Can you work these out from the model? Positions are in its coordinate system, mm. Face numbers are marked on the shaded views. A direction names the side the tool comes from. Give positions to 0.01 mm unless a question says otherwise; leave off trailing zeros. Write each loop counter-clockwise with the first axis right and the second up, starting at its lowest first coordinate (ties: lowest second). Pieces come first, ordered by that corner, then holes. Notation, with made-up numbers: M 85.25,62.25 L 140.25,62.25 A21 cw 140.25,70.25 Z; hole C 10.25,-4.5 d10. An arc over 180 degrees is marked long. Use CSV: the item, a comma, the result in double quotes. Start each with the question number.
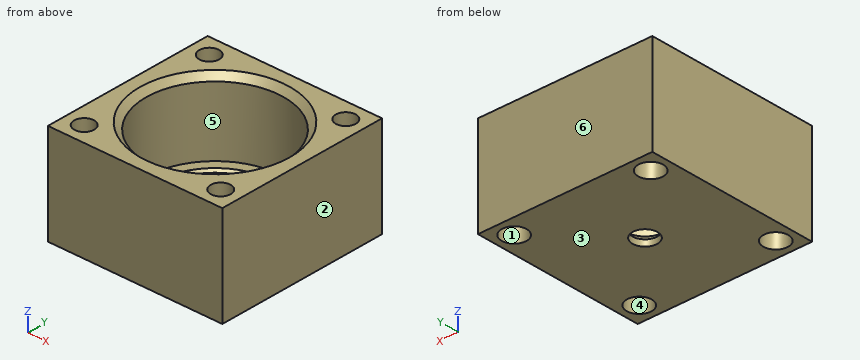
from build123d import *

# Parameters (mm, degrees)
SKETCH_W        = 28
SKETCH_H        = 28
SKETCH_R        = 2
PAD_DEPTH       = 2
SKETCH001_W     = 28
SKETCH001_H     = 28
SKETCH001_R     = 9
SKETCH001_R_2   = 2
PAD001_DEPTH    = 2
SKETCH003_W     = 28
SKETCH003_H     = 28
SKETCH003_R     = 1.6
SKETCH003_R_2   = 11
PAD002_DEPTH    = 12
CHAMFER_SIZE    = 1
CHAMFER001_SIZE = 0.4
CHAMFER002_SIZE = 1


with BuildPart() as part:
    # Sketch → Pad (new body)
    with BuildSketch(Plane.XY):
        Rectangle(SKETCH_W, SKETCH_H)
        Circle(SKETCH_R, mode=Mode.SUBTRACT)
        with Locations((10.960155, 10.960155)):
            Circle(SKETCH_R, mode=Mode.SUBTRACT)
        with Locations((-10.960155, 10.960155)):
            Circle(SKETCH_R, mode=Mode.SUBTRACT)
        with Locations((-10.960155, -10.960155)):
            Circle(SKETCH_R, mode=Mode.SUBTRACT)
        with Locations((10.960155, -10.960155)):
            Circle(SKETCH_R, mode=Mode.SUBTRACT)
    extrude(amount=PAD_DEPTH)

    # Sketch001 (on Face11 of Pad) → Pad001 (join)
    with BuildSketch(Plane.XY.offset(2)):
        Rectangle(SKETCH001_W, SKETCH001_H)
        Circle(SKETCH001_R, mode=Mode.SUBTRACT)
        with Locations((-10.960155, 10.960155)):
            Circle(SKETCH001_R_2, mode=Mode.SUBTRACT)
        with Locations((-10.960155, -10.960155)):
            Circle(SKETCH001_R_2, mode=Mode.SUBTRACT)
        with Locations((10.960155, -10.960155)):
            Circle(SKETCH001_R_2, mode=Mode.SUBTRACT)
        with Locations((10.960155, 10.960155)):
            Circle(SKETCH001_R_2, mode=Mode.SUBTRACT)
    extrude(amount=PAD001_DEPTH)

    # Sketch003 (on Face14 of Pad001) → Pad002 (join)
    with BuildSketch(Plane.XY.offset(4)):
        Rectangle(SKETCH003_W, SKETCH003_H)
        with Locations((-10.960155, 10.960155)):
            Circle(SKETCH003_R, mode=Mode.SUBTRACT)
        with Locations((-10.960155, -10.960155)):
            Circle(SKETCH003_R, mode=Mode.SUBTRACT)
        with Locations((10.960155, -10.960155)):
            Circle(SKETCH003_R, mode=Mode.SUBTRACT)
        with Locations((10.960155, 10.960155)):
            Circle(SKETCH003_R, mode=Mode.SUBTRACT)
        Circle(SKETCH003_R_2, mode=Mode.SUBTRACT)
    extrude(amount=PAD002_DEPTH)

    # Chamfer
    chamfer_edges = [part.edges().sort_by_distance(p)[0] for p in [
        (-11, 0, 16),
    ]]
    chamfer(chamfer_edges, length=CHAMFER_SIZE)

    # Chamfer001
    chamfer001_edges = [part.edges().sort_by_distance(p)[0] for p in [
        (-9, 0, 4),
    ]]
    chamfer(chamfer001_edges, length=CHAMFER001_SIZE)

    # Chamfer002
    chamfer002_edges = [part.edges().sort_by_distance(p)[0] for p in [
        (-2, 0, 2),
    ]]
    chamfer(chamfer002_edges, length=CHAMFER002_SIZE)


solid = part.part
(1) Which directions (+Z, -Z, +X, -X, +Y, -Y) give clear straight access to the entire face, cutting with the end or side of a thin tool? Please do the marked faces 4, 5 and 6.
(2) Thinking about a two-plate mould opening in X: for the marked faces 1, 2 and 3, which applies, released by +X, released by -X, zero draft, split by the parting line, or undercut?
(3) I want a section at C-C (z = 8.5). Write out the boundary of the cut face in (x, y).
(4) I want a section at D-D (y = -10.5). State how many separate pieces and enclosed holes the cut face has, and give its area (3 significant figures).
(5) Will these pins go through, and if not, where does the flat tip stop? pin 1 Ø1 at (x, y) = (-4, 1) entering from +Z; pin 2 Ø2 at (x, y) = (-10.5, -10.5) entering from -Z; pin 3 Ø4 at (x, y) = (-7.5, -1) entering from +Z; pin 4 Ø2 at (x, y) = (11, 10.5) entering from -Z.
(6) Please list where these lines run through material, in increasing order: L1, parallel to Y at x = 0, z = 6.25; L2, parallel to Y at x = 0, z = 0.6; L3, parallel to Z at x = -5.5, y = 8.25. Write a range as [from, to].
(7) I want a section at A-A (x = 0). Write out the boundary of the cut face in (y, z).
Geometry results:
1,face 4,"-Z"
1,face 5,"+Z"
1,face 6,"+Z, -Z, +X, -X, +Y"
2,face 1,"undercut"
2,face 2,"released by +X"
2,face 3,"zero draft"
3,outline,"M -14,-14 L 14,-14 L 14,14 L -14,14 Z; hole C -10.96,-10.96 d3.2; hole C -10.96,10.96 d3.2; hole C 0,0 d22; hole C 10.96,-10.96 d3.2; hole C 10.96,10.96 d3.2"
4,separate pieces,"3"
4,enclosed holes,"0"
4,area,"262 mm2"
5,pin 1,"stops at z = 2"
5,pin 2,"stops at z = 4"
5,pin 3,"stops at z = 4"
5,pin 4,"passes through"
6,L1,"y = [-14, -11], [11, 14]"
6,L2,"y = [-14, -2], [2, 14]"
6,L3,"z = [0, 4]"
7,outline,"M -14,0 L -2,0 L -2,1 L -3,2 L -9,2 L -9,3.6 L -9.4,4 L -11,4 L -11,15 L -12,16 L -14,16 Z; M 2,0 L 14,0 L 14,16 L 12,16 L 11,15 L 11,4 L 9.4,4 L 9,3.6 L 9,2 L 3,2 L 2,1 Z"
